Geometry: final body of the model. Coordinates: model frame, mm. A direction names the side the tool comes from. Coordinates: 2 decimals unless noted, no trailing zeros. Write each loop counter-clockwise with the first axis right and the second up, starting at its lowest first coordinate (ties: lowest second). Pieces come first, ordered by that corner, then holes. Notation, with made-up numbers: (74, 67) - (120, 67) arc R17 ccw to (120, 76) - close; hole circle Ø10 at (28.5, 11.25). An arc over 180 degrees is marked (long way). Answer as a JSON object with one key per item and string values. Group by question number.
Item 1: Line query: line 1 along X through (y, z) = (0.3, -3); line 2 along Z through (x, y) = (-11.5, -0.3). Output: solid intervals per line, ascending. Write a range as from..to.
Item 2: Section D-D on z = 21.5. Return loops of the section in (x, y), and give its area (3 significant figures).
Item 3: Section A-A on z = -3.5. Return loops of the section in (x, y), and give its area (3 significant figures).
Item 4: First-contact query: pin 1 Ø0.8 at (y, z) = (1, -46) entering from -X; pin 2 Ø1.2 at (y, z) = (1.5, -44) entering from +X; pin 3 Ø2 at (x, y) = (-47.5, 1.5) entering from -Z. Flat tips, straight axial feed; report the tip coordinate or a pass-through.
Item 5: Mould query, pull axis Z, two halves, no side actions, for faces 4 (the flat face through (32.5, -1, 0)), 5 (the flat face through (46, 1, -12.37)), 6 (the flat face through (0, 2.5, -46)), 7 (the flat face through (0, -1, 32.5)). Classes: pulls with the +Z half, pulls with the -Z half, needs draft (parallel to the pull), parting line crosses it, or undercut.
Item 6: Set-up query: faces 1 (the flat face through (41.389, 1, 0)), 2 (the flat face through (12.37, 1, -46)), 3 (the flat face through (0, 1, -41.25)). Return all of +Z, -Z, +X, -X, +Y, -Y with unobstructed straight access to the full face (end or side cutting, diameter ignored); none if empty.
Item 7: Section C-C on x = 8.5. Return loops of the section in (y, z).
Item 8: Section B-B on y = -0.8. Return loops of the section in (x, z).
```python
from build123d import *

# Parameters (mm, degrees)
F0_W     = 100
F0_H     = 100
F0_W_2   = 65
F0_H_2   = 65
F1_DEPTH = 2.5
F2_W     = 8.75
F2_H     = 24.739
F3_DEPTH = 2.5
F4_W     = 8.61061
F4_H     = 24.739
F5_DEPTH = 2.5
F6_W     = 24.739
F6_H     = 2.5
F7_DEPTH = 8.75


with BuildPart() as f1:
    # F0 (on Front) → F1 (new body)
    with BuildSketch(Plane.XZ):
        Rectangle(F0_W, F0_H)
        Rectangle(F0_W_2, F0_H_2, mode=Mode.SUBTRACT)
    extrude(amount=F1_DEPTH)

    # F2 (on face) → F3 (join)
    with BuildSketch(Plane(origin=(0, 0, 0), x_dir=(-1, 0, 0), z_dir=(0, 1, 0))):
        with Locations((45.625, -0.188954)):
            Rectangle(F2_W, F2_H)
    extrude(amount=F3_DEPTH)

    # F4 (on face) → F5 (join)
    with BuildSketch(Plane(origin=(0, 0, 0), x_dir=(-1, 0, 0), z_dir=(0, 1, 0))):
        with Locations((-45.694695, 0)):
            Rectangle(F4_W, F4_H)
    extrude(amount=F5_DEPTH)

    # F6 (on face) → F7 (join)
    with BuildSketch(Plane(origin=(0, 0, -50), x_dir=(1, 0, 0), z_dir=(0, 0, -1))):
        with Locations((0, -1.25)):
            Rectangle(F6_W, F6_H)
    extrude(amount=-F7_DEPTH)


solid = f1.part
```
Checks:
{
 "1": {"line 1": "-50..-41.25, 41.39..50", "line 2": "-50..-32.5, 32.5..50"},
 "2": {"outline": "(-50, -2.5) - (-32.5, -2.5) - (-32.5, 0) - (-50, 0) - close; (32.5, -2.5) - (50, -2.5) - (50, 0) - (32.5, 0) - close", "area": "87.5 mm^2"},
 "3": {"outline": "(-50, -2.5) - (-32.5, -2.5) - (-32.5, 0) - (-41.25, 0) - (-41.25, 2.5) - (-50, 2.5) - close; (32.5, -2.5) - (50, -2.5) - (50, 2.5) - (41.39, 2.5) - (41.39, 0) - (32.5, 0) - close", "area": "131 mm^2"},
 "4": {"pin 1": "x = -12.37", "pin 2": "x = 12.37", "pin 3": "z = -12.56"},
 "5": {"face 4": "undercut", "face 5": "pulls with the -Z half", "face 6": "needs draft", "face 7": "undercut"},
 "6": {"face 1": "+Z, -Z, +Y", "face 2": "+Z, -Z, +X, +Y", "face 3": "+Z, +X, -X, +Y"},
 "7": {"outline": "(-2.5, -50) - (2.5, -50) - (2.5, -41.25) - (0, -41.25) - (0, -32.5) - (-2.5, -32.5) - close; (-2.5, 32.5) - (0, 32.5) - (0, 50) - (-2.5, 50) - close"},
 "8": {"outline": "(-50, -50) - (50, -50) - (50, 50) - (-50, 50) - close; hole (-32.5, -32.5) - (32.5, -32.5) - (32.5, 32.5) - (-32.5, 32.5) - close"}
}
